For this review, take the finished solid that the model builds, in its own axes (mm). Face numbers are marked on the shaded views. Round coordinates to 2 decimals unless told otherwise and drop trailing zeros. Loops run counter-clockwise (first coordinate to the right, second up) from the corner with the lowest first, then second, coordinate; pieces in that order, holes last. Notation, with made-up numbers: (70.5, 30.5) -> (85.5, 30.5) arc R27 ccw to (85.5, 62.5) -> close; hole circle Ø2 at (43, 63.5). An arc over 180 degrees is marked (long way). Use one line per item in the form item = value. Start each with the question number.
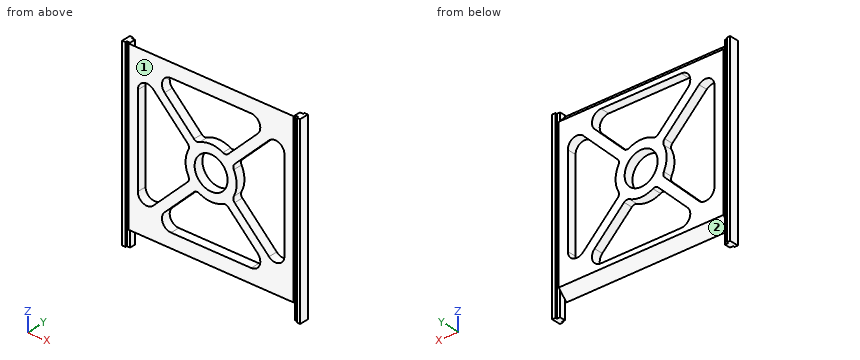
from build123d import *

# Parameters (mm, degrees)
BOSS_EXTRUDE1_DEPTH = 5.5
SKETCH4_W           = 2
SKETCH4_H           = 1
CUT_EXTRUDE2_DEPTH  = 110
SKETCH5_R           = 10
CUT_EXTRUDE3_DEPTH  = 110
CUT_EXTRUDE4_START  = -4
CUT_EXTRUDE4_DEPTH  = 100
FILLET3_R           = 5.5
FILLET4_R           = 2.75


with BuildPart() as part:
    # Sketch1 → Boss-Extrude1 (new body)
    with BuildSketch(Plane(origin=(0, 0, 0), x_dir=(1, 0, 0), z_dir=(0, 1, 0))):
        Polygon((0, 110), (4, 110), (4, 100), (104, 100), (104, 110), (108, 110), (108, 0), (0, 0), align=None)
    extrude(amount=BOSS_EXTRUDE1_DEPTH)

    # Sketch4 → Cut-Extrude2 (cut)
    with BuildSketch(Plane(origin=(0, 0, -110), x_dir=(-1, 0, 0), z_dir=(0, 0, -1))):
        with Locations((-3, 0.5)):
            Rectangle(SKETCH4_W, SKETCH4_H)
        with Locations((-3, 5)):
            Rectangle(SKETCH4_W, SKETCH4_H)
        with Locations((-105, 5)):
            Rectangle(SKETCH4_W, SKETCH4_H)
        with Locations((-105, 0.5)):
            Rectangle(SKETCH4_W, SKETCH4_H)
    extrude(amount=-CUT_EXTRUDE2_DEPTH, mode=Mode.SUBTRACT)

    # Sketch5 → Cut-Extrude3 (cut)
    with BuildSketch(Plane(origin=(0, 5.5, 0), x_dir=(1, 0, 0), z_dir=(0, 1, 0))):
        with Locations(Location((54, 50, 0), (0, 0, 270))):
            Circle(SKETCH5_R)
        with BuildLine():
            Line((41.269180349, 41.158267646), (9.5, 9.389087297))
            Line((9.5, 9.389087297), (9.5, 90.610912703))
            Line((9.5, 90.610912703), (41.269180349, 58.841732354))
            ThreePointArc((41.269180349, 58.841732354), (38.5, 50), (41.269180349, 41.158267646))
        make_face()
        with BuildLine():
            Line((98.5, 90.610912703), (98.5, 9.389087297))
            Line((98.5, 9.389087297), (66.730819651, 41.158267646))
            ThreePointArc((66.730819651, 41.158267646), (69.5, 50), (66.730819651, 58.841732354))
            Line((66.730819651, 58.841732354), (98.5, 90.610912703))
        make_face()
        with BuildLine():
            Line((45.158267646, 62.730819651), (16.389087297, 91.5))
            Line((16.389087297, 91.5), (91.610912703, 91.5))
            Line((91.610912703, 91.5), (62.841732354, 62.730819651))
            ThreePointArc((62.841732354, 62.730819651), (54, 65.5), (45.158267646, 62.730819651))
        make_face()
        with BuildLine():
            Line((16.389087297, 8.5), (91.610912703, 8.5))
            Line((91.610912703, 8.5), (62.841732354, 37.269180349))
            ThreePointArc((62.841732354, 37.269180349), (54, 34.5), (45.158267646, 37.269180349))
            Line((45.158267646, 37.269180349), (16.389087297, 8.5))
        make_face()
    extrude(amount=-CUT_EXTRUDE3_DEPTH, mode=Mode.SUBTRACT)

    # Sketch6 → Cut-Extrude4 (cut)
    with BuildSketch(Plane(origin=(108, 0, 0), x_dir=(0, 0, -1), z_dir=(1, 0, 0)).offset(CUT_EXTRUDE4_START)):
        Polygon((0, 0), (5.5, 5.5), (0, 5.5), align=None)
        Polygon((100, 5.5), (100, 0), (94.5, 5.5), align=None)
    extrude(amount=-CUT_EXTRUDE4_DEPTH, mode=Mode.SUBTRACT)

    # Fillet3
    fillet3_edges = [part.edges().sort_by_distance(p)[0] for p in [
        (16.389087297, 2.75, -91.5),
        (91.610912703, 2.75, -91.5),
        (9.5, 2.75, -9.389087297),
        (9.5, 2.75, -90.610912703),
        (98.5, 2.75, -90.610912703),
        (98.5, 2.75, -9.389087297),
        (16.389087297, 2.75, -8.5),
        (91.610912703, 2.75, -8.5),
    ]]
    fillet(fillet3_edges, radius=FILLET3_R)

    # Fillet4
    fillet4_edges = [part.edges().sort_by_distance(p)[0] for p in [
        (62.841732354, 2.75, -62.730819651),
        (45.158267646, 2.75, -62.730819651),
        (41.269180349, 2.75, -58.841732354),
        (41.269180349, 2.75, -41.158267646),
        (66.730819651, 2.75, -41.158267646),
        (66.730819651, 2.75, -58.841732354),
        (45.158267646, 2.75, -37.269180349),
        (62.841732354, 2.75, -37.269180349),
    ]]
    fillet(fillet4_edges, radius=FILLET4_R)


solid = part.part
Item 1: Wall thickness on line 1 (X direction, y = 4.35, z = -50); line 2 (X direction, y = 1.05, z = -14.5); line 3 (Z direction, x = 53.5, y = 5.05): over which ranges is each line inside the solid? List them lowest first.
Item 2: Take a section at C-C on x = 66. Give the boundary of the cut face in (y, z), plus the area to 3 significant figures.
Item 3: Draft analysis for pull direction X (two halves, no side actions). For the marked faces 1 and 2, state which applies: +X half, -X half, draft (parallel to the pull), parting line (faces both ways), or undercut.
Item 4: For P1, Ø12, axis at x = 54, z = -50, coming from the +Y side; P2, Ø1, axis at x = 105, z = -53.5, coming from the +Y side; P3, Ø0.6, axis at x = 105, z = -49, coming from the -Y side; P4, Ø1.6, axis at x = 62.5, y = 4, coming from the -Z side, all flat-tipped, find the tip position at first contact; note any pin that passes through.
Item 5: Take a section at A-A on z = -50. Give the number of separate pieces and of enclosed holes in the cut face, plus the area to 3 significant figures.
Item 6: Take a section at B-B on x = 54. Give the boundary of the cut face in (y, z), plus the area to 3 significant figures.
Results:
q1.line_1 = 0 to 9.5, 38.5 to 44, 64 to 69.5, 98.5 to 108
q1.line_2 = 0 to 24.19, 83.81 to 108
q1.line_3 = -94.95 to -91.5, -65.49 to -59.99, -40.01 to -34.51, -8.5 to -5.05
q2.outline = (0, -100) -> (5.5, -94.5) -> (5.5, -91.5) -> (0, -91.5) -> close; (0, -65.89) -> (5.5, -65.89) -> (5.5, -34.11) -> (0, -34.11) -> close; (0, -8.5) -> (5.5, -8.5) -> (5.5, -5.5) -> (0, 0) -> close
q2.area = 238 mm2
q3.face_1 = draft
q3.face_2 = undercut
q4.P1 = through
q4.P2 = 4.5
q4.P3 = 1
q4.P4 = -96.8
q5.separate_pieces = 4
q5.enclosed_holes = 0
q5.area = 157 mm2
q6.outline = (0, -100) -> (5.5, -94.5) -> (5.5, -91.5) -> (0, -91.5) -> close; (0, -65.5) -> (5.5, -65.5) -> (5.5, -60) -> (0, -60) -> close; (0, -40) -> (5.5, -40) -> (5.5, -34.5) -> (0, -34.5) -> close; (0, -8.5) -> (5.5, -8.5) -> (5.5, -5.5) -> (0, 0) -> close
q6.area = 124 mm2
